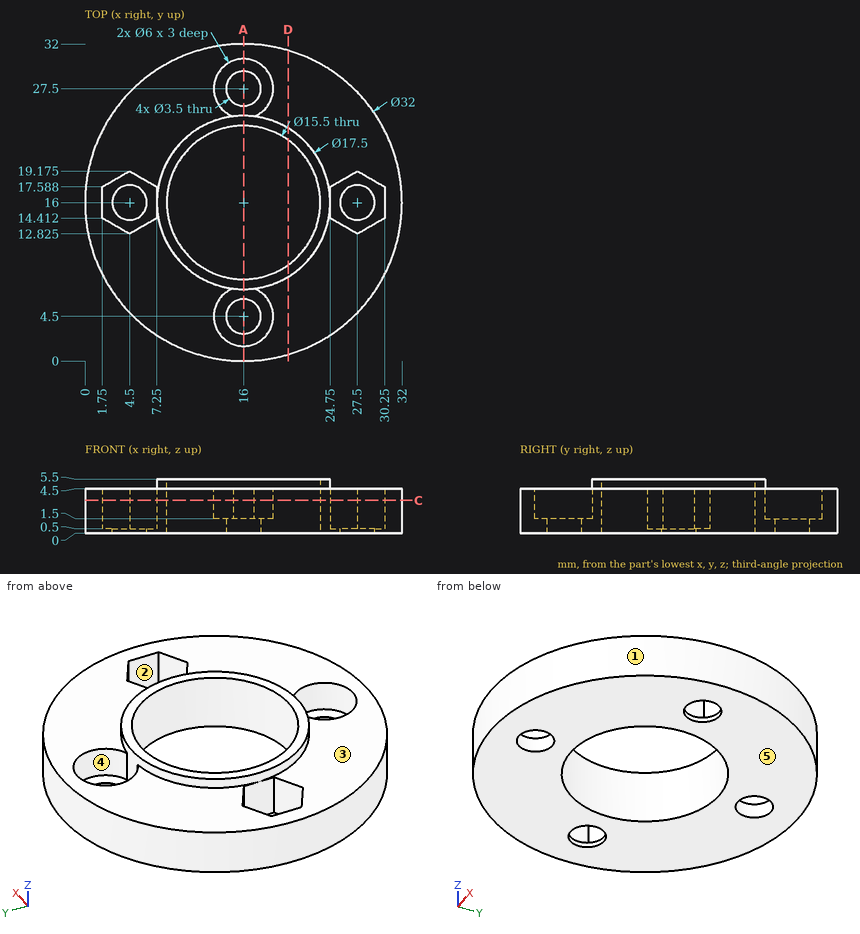
Verification items for this drawing (mm, ordinates from the low corner). A direction names the side the tool comes from. Coordinates: 2 decimals unless noted, no trailing zeros. Loops run counter-clockwise (first coordinate to the right, second up) from the corner with the lowest first, then second, coordinate; pieces in that order, holes last. Notation, with made-up numbers: (80, 54.25) - (130, 54.25) arc R31 ccw to (130, 79.25) - close; hole circle Ø7 at (65, -25.5). An arc over 180 degrees is marked (long way). Answer as a JSON object with one key per item and string values.
(1) Access from +Z, -Z, +X, -X, +Y, -Y to the whole of each face (thin tool, end or side, straight path). Record for the marked faces 4 and 5.
Response:
{"face 4": "+Z", "face 5": "-Z, +X, -X, +Y, -Y"}
(2) Cross-section at A-A, the plane x = 16. Record the boundary of the cut face in (y, z).
Response:
{"outline": "(0, 0) - (2.75, 0) - (2.75, 1.5) - (1.5, 1.5) - (1.5, 4.5) - (0, 4.5) - close; (6.25, 0) - (8.25, 0) - (8.25, 5.5) - (7.25, 5.5) - (7.25, 1.5) - (6.25, 1.5) - close; (23.75, 0) - (25.75, 0) - (25.75, 1.5) - (24.75, 1.5) - (24.75, 5.5) - (23.75, 5.5) - close; (29.25, 0) - (32, 0) - (32, 4.5) - (30.5, 4.5) - (30.5, 1.5) - (29.25, 1.5) - close"}
(3) Cross-section at C-C, the plane z = 3.35. Count the separate pieces of the cut face and the enclosed holes in it, then the cut area to 3 significant figures.
Response:
{"separate pieces": "1", "enclosed holes": "5", "area": "507 mm²"}
(4) Scan lines: line 1 along Y through (x, z) = (16, 0.75); line 2 along Y through (x, z) = (16.5, 4) (1 decimal); line 3 along Z through (x, y) = (4.5, 11.5). Record each from-to range of solid material in increasing order.
Response:
{"line 1": "y = 0 to 2.75, 6.25 to 8.25, 23.75 to 25.75, 29.25 to 32", "line 2": "y = 0 to 1.5, 7.3 to 8.3, 23.7 to 24.7, 30.5 to 32", "line 3": "z = 0 to 4.5"}
(5) Cross-section at D-D, the plane x = 20.5. Record the boundary of the cut face in (y, z).
Response:
{"outline": "(0.65, 0) - (9.69, 0) - (9.69, 5.5) - (8.5, 5.5) - (8.5, 4.5) - (0.65, 4.5) - close; (22.31, 0) - (31.35, 0) - (31.35, 4.5) - (23.5, 4.5) - (23.5, 5.5) - (22.31, 5.5) - close"}
(6) Mould release check, pull along Y, two halves, no side actions. Record for the marked faces 1, 2 and 3: pulls with the +Y half, pulls with the -Y half, needs draft (parallel to the pull), parting line crosses it, or undercut.
Response:
{"face 1": "parting line crosses it", "face 2": "undercut", "face 3": "needs draft"}
(7) Go/stop test with flat-tipped pins: pin 1 Ø3 at (x, z) = (20.5, 1.5) entering from -Y; pin 2 Ø1 at (x, z) = (10.5, 3) entering from -Y; pin 3 Ø3 at (x, y) = (17.5, 27) entering from +Z. Record where each tip stops, or that it passes through.
Response:
{"pin 1": "stops at y = 0.28", "pin 2": "stops at y = 0.8", "pin 3": "stops at z = 4.5"}
